from build123d import *

# Parameters (mm, degrees)
F0_R     = 4
F1_DEPTH = 8


with BuildPart() as f1:
    # F0 (on Front) → F1 (new body)
    with BuildSketch(Plane.XZ):
        with BuildLine():
            Line((-10, 29.910809), (-10, 0))
            ThreePointArc((-10, 0), (0, -10), (10, 0))
            Line((10, 0), (10, 29.910809))
            Line((10, 29.910809), (10, 30.089191))
            ThreePointArc((10, 30.089191), (-0.089191, 40), (-10, 29.910809))
        make_face()
        Circle(F0_R, mode=Mode.SUBTRACT)
        with Locations((0, 30)):
            Circle(F0_R, mode=Mode.SUBTRACT)
        with BuildLine():
            Line((10, 30.089191), (10, 29.910809))
            ThreePointArc((10, 29.910809), (10.000398, 30), (10, 30.089191))
        make_face()
    extrude(amount=F1_DEPTH)


solid = f1.part
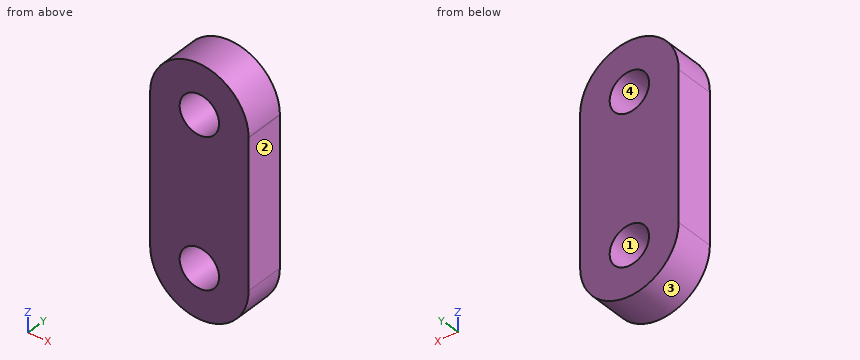
Check sheet for the modelled part. Datum: model origin and axes. Units: mm. Face numbers are marked on the shaded views. Round coordinates to 2 decimals unless told otherwise and drop trailing zeros. Order: outer loops, then holes, each group sorted by start corner. A loop starts at its lowest first (then second) coordinate and runs counter-clockwise, first axis right, second up. Notation, with made-up numbers: M 6,72.5 L 33,72.5 A5 cw 33,79.5 Z; hole C 73,31 d6. An arc over 180 degrees is marked long. One line per item, written item: value. Start each with the question number.
1. Gauge pin test, flat ends, axial feed: P1, Ø1, axis at x = -4, y = -1.5, coming from the -Z side; P2, Ø1.5, axis at y = -5, z = 33.5, coming from the +X side. Record the tip position at first contact, or that the pin passes through.
2. Release check for a two-part mould opening along Z. For the marked faces 1, 2, 3 and 4 record: released by +Z, released by -Z, zero draft, split by the parting line, or undercut.
3. Section check B-B on y = -6. Enter the section's corners in (x, z).
4. Section check C-C on z = 26.5. Enter the section's corners in (x, y), and give its area (3 significant figures).
5. Scan lines: line 1 along Z through (x, y) = (0, -3.75); line 2 along Z through (x, y) = (-1.25, -3.75); line 3 along X through (y, z) = (-2.75, 29.5). Record each from-to range of solid material in increasing order.
6. Section check A-A on x = 0. Enter the section's corners in (y, z).
7. Section check D-D on x = 2.25. Enter the section's corners in (y, z).
Results found:
1. P1: z = -9.37
1. P2: x = 9.61
2. face 1: undercut
2. face 2: zero draft
2. face 3: released by -Z
2. face 4: undercut
3. outline: M -10,0 A10 ccw 10,0 L 10,29.91 A9.99 ccw 10,30.09 A10 ccw -10,29.91 Z; hole C 0,0 d8; hole C 0,30 d8
4. outline: M -10,-8 L -1.94,-8 L -1.94,0 L -10,0 Z; M 1.94,-8 L 10,-8 L 10,0 L 1.94,0 Z
4. area: 129 mm^2
5. line 1: -10 to -4, 4 to 26, 34 to 40
5. line 2: -9.92 to -3.8, 3.8 to 26.2, 33.8 to 39.92
5. line 3: -10 to -3.97, 3.97 to 10
6. outline: M -8,-10 L 0,-10 L 0,-4 L -8,-4 Z; M -8,4 L 0,4 L 0,26 L -8,26 Z; M -8,34 L 0,34 L 0,40 L -8,40 Z
7. outline: M -8,-9.74 L 0,-9.74 L 0,-3.31 L -8,-3.31 Z; M -8,3.31 L 0,3.31 L 0,26.69 L -8,26.69 Z; M -8,33.31 L 0,33.31 L 0,39.74 L -8,39.74 Z
